The model under review builds one solid part; all positions refer to its coordinate system, in mm. Face numbers are marked on the shaded views. A direction names the side the tool comes from. Coordinates: 2 decimals unless noted, no trailing zeros. Order: outer loops, then holes, each group sorted by start corner. A loop starts at its lowest first (then second) coordinate and runs counter-clockwise, first axis right, second up. Notation, with made-up numbers: (43, -34.75) -> (95, -34.75) arc R24 cw to (95, 4.25) -> close; hole circle Ø6 at (36, 79.5). An arc over 180 degrees is marked (long way). Use one line per item in the form item = value. Start each with the question number.
(1) Take a section at A-A (y = 9.5). State how many separate pieces and enclosed holes the cut face has, then the cut area to 3 significant figures.
(2) Take a section at B-B (z = 4.2). State the section outline as (x, y) points.
(3) Mouldability with a two-part tool opening along X and no side actions: class the marked faces 1, 2 and 3 as +X half, -X half, draft (parallel to the pull), parting line (faces both ways), or undercut.
(4) Wall thickness on line 1 along Z through (x, y) = (0, 6.75); line 2 along Y through (x, z) = (5, 0.65); line 3 along Y through (x, z) = (9.5, 1.25): over which ranges is each line inside the solid? List them lowest first.
(5) For the marked faces 4 and 5, list the 3-axis set-ups (+Z, -Z, +X, -X, +Y, -Y) from which the entire face can be reached by the end or side of a thin tool; tool diameter is ignored.
(6) Insertion check: pin 1 Ø2 at (x, z) = (3.5, 14.5) entering from -Y; pin 2 Ø2 at (y, z) = (6.5, 32.5) entering from +X; pin 3 Ø14 at (x, y) = (2, -8) entering from +Z. Each pin has a flat end and moves straight along its axis. Give the tip position at first contact, or say it passes through.
```python
from build123d import *

# Parameters (mm, degrees)
SKETCH1_W           = 33
SKETCH1_H           = 28
BOSS_EXTRUDE1_DEPTH = 46
CUT_EXTRUDE1_DEPTH  = 46
CUT_EXTRUDE2_START  = -3
CUT_EXTRUDE2_DEPTH  = 27
FILLET2_R           = 12.5
FILLET3_R           = 16.5
FILLET4_R           = 6
SKETCH4_W           = 13
SKETCH4_H           = 23
CUT_EXTRUDE3_DEPTH  = 9
SKETCH5_R           = 6.5
CUT_EXTRUDE4_DEPTH  = 56.592265809
SKETCH6_R           = 1
CUT_EXTRUDE5_DEPTH  = 8
SKETCH7_R           = 1.3
SKETCH7_R_2         = 2.5
CUT_EXTRUDE6_DEPTH  = 1.769084801


with BuildPart() as part:
    # Sketch1 → Boss-Extrude1 (new body)
    with BuildSketch(Plane.XY):
        Rectangle(SKETCH1_W, SKETCH1_H)
    extrude(amount=BOSS_EXTRUDE1_DEPTH)

    # Sketch2 → Cut-Extrude1 (cut)
    with BuildSketch(Plane(origin=(16.5, 0, 0), x_dir=(0, 0, -1), z_dir=(1, 0, 0))):
        with BuildLine():
            Line((-46, 2), (-46, -14))
            Line((-46, -14), (-5, -14))
            add(Edge.make_bspline(
                [(-5, -14), (-24.751807392, -3.724011785), (-46, 2)],
                knots=[0, 0, 0, 1, 1, 1], degree=2))
        make_face()
    extrude(amount=-CUT_EXTRUDE1_DEPTH, mode=Mode.SUBTRACT)

    # Sketch3 → Cut-Extrude2 (cut)
    with BuildSketch(Plane(origin=(16.5, 0, 0), x_dir=(0, 0, -1), z_dir=(1, 0, 0)).offset(CUT_EXTRUDE2_START)):
        with BuildLine():
            Line((-5, -14), (-1.769084801, -14))
            Line((-1.769084801, -14), (-1.769084801, 3.5))
            Line((-1.769084801, 3.5), (-39.769084801, 3.5))
            Line((-39.769084801, 3.5), (-39.769084801, 0.213825967))
            add(Edge.make_bspline(
                [(-5, -14), (-21.840644779, -5.238560409), (-39.769084801, 0.213825967)],
                knots=[0, 0, 0, 1, 1, 1], degree=2))
        make_face()
    extrude(amount=-CUT_EXTRUDE2_DEPTH, mode=Mode.SUBTRACT)

    # Fillet2
    fillet2_edges = [part.edges().sort_by_distance(p)[0] for p in [
        (13.5, 1.856912984, 39.769084801),
        (-13.5, 1.856912984, 39.769084801),
    ]]
    fillet(fillet2_edges, radius=FILLET2_R)

    # Fillet3
    fillet3_edges = [part.edges().sort_by_distance(p)[0] for p in [
        (16.5, 8, 46),
        (-16.5, 8, 46),
    ]]
    fillet(fillet3_edges, radius=FILLET3_R - 0.0001)  # a hair under: the kernel refuses the full size

    # Fillet4
    fillet4_edges = [part.edges().sort_by_distance(p)[0] for p in [
        (-16.5, -14, 2.5),
        (16.5, -14, 2.5),
    ]]
    fillet(fillet4_edges, radius=FILLET4_R)

    # Sketch4 → Cut-Extrude3 (cut)
    with BuildSketch(Plane.XZ.offset(-3.5)):
        with Locations((0, 18)):
            Rectangle(SKETCH4_W, SKETCH4_H)
    extrude(amount=-CUT_EXTRUDE3_DEPTH, mode=Mode.SUBTRACT)

    # Sketch5 → Cut-Extrude4 (cut, through all)
    with BuildSketch(Plane.XZ.offset(-12.5)):
        with Locations((0, 23)):
            Circle(SKETCH5_R)
    extrude(amount=-CUT_EXTRUDE4_DEPTH, mode=Mode.SUBTRACT)

    # Sketch6 → Cut-Extrude5 (cut)
    with BuildSketch(Plane.XZ.offset(-3.5)):
        with Locations((0, 31.8)):
            Circle(SKETCH6_R)
        with Locations((0, 4.2)):
            Circle(SKETCH6_R)
    extrude(amount=-CUT_EXTRUDE5_DEPTH, mode=Mode.SUBTRACT)

    # Sketch7 → Cut-Extrude6 (cut)
    with BuildSketch(Plane(origin=(0, 0, 0), x_dir=(-1, 0, 0), z_dir=(0, 0, -1))):
        with Locations((-9.5, 0)):
            Circle(SKETCH7_R)
        with Locations((-5, 0)):
            Circle(SKETCH7_R_2)
        with Locations((-0.5, 0)):
            Circle(SKETCH7_R)
    extrude(amount=-CUT_EXTRUDE6_DEPTH, mode=Mode.SUBTRACT)


solid = part.part
```
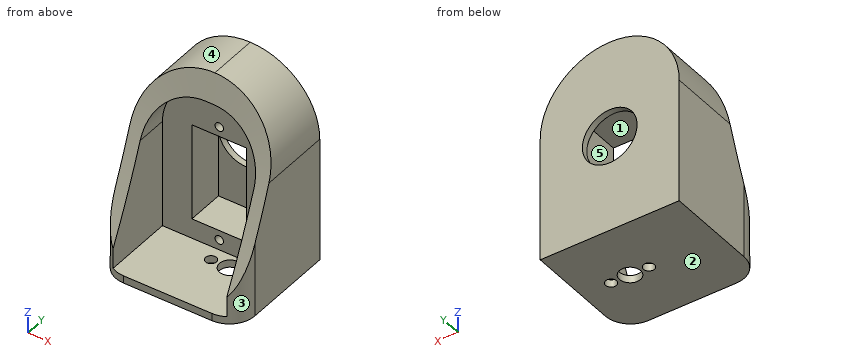
Findings:
q1.separate_pieces = 1
q1.enclosed_holes = 3
q1.area = 1,100 mm²
q2.outline = (-16.5, -8) arc R6 ccw to (-13.5, -13.2) -> (-13.5, 3.5) -> (-1, 3.5) -> (-1, 11.5) -> (1, 11.5) -> (1, 3.5) -> (13.5, 3.5) -> (13.5, -13.2) arc R6 ccw to (16.5, -8) -> (16.5, 14) -> (-16.5, 14) -> close
q3.face_1 = undercut
q3.face_2 = draft
q3.face_3 = +X half
q4.line_1 = 0 to 3.2, 5.2 to 6.5, 29.5 to 30.8, 32.8 to 46
q4.line_2 = -14 to -2.5, 2.5 to 14
q4.line_3 = -14 to -1.3, 1.3 to 14
q5.face_4 = +Z, -X, +Y, -Y
q5.face_5 = -Y
q6.pin_1 = 12.5
q6.pin_2 = 16.38
q6.pin_3 = 1.77
